Verification items for the finished model (mm, model axes). A direction names the side the tool comes from. Round coordinates to 2 decimals unless told otherwise and drop trailing zeros. Write each loop counter-clockwise with the first axis right and the second up, starting at its lowest first coordinate (ties: lowest second). Pieces come first, ordered by that corner, then holes. Notation, with made-up numbers: (64.5, -20.5) - (98.5, -20.5) arc R9 ccw to (98.5, -4.5) - close; hole circle Ø9 at (33, 44.5). An arc over 180 degrees is marked (long way). Answer as a JSON object with one key per item and string values.
```python
from build123d import *

# Parameters (mm, degrees)
BOSS_EXTRUDE1_DEPTH = 10
BOSS_EXTRUDE2_DEPTH = 130
FILLET1_R           = 0.8
SKETCH3_R           = 20
CUT_EXTRUDE1_DEPTH  = 5
CUT_EXTRUDE2_DEPTH  = 2


with BuildPart() as part:
    # Sketch1 → Boss-Extrude1 (new body)
    with BuildSketch(Plane(origin=(0, 0, 0), x_dir=(1, 0, 0), z_dir=(0, 1, 0))):
        Polygon((-35, 30), (-30, 35), (30, 35), (35, 30), (35, -30), (30, -35), (-30, -35), (-35, -30), align=None)
    extrude(amount=BOSS_EXTRUDE1_DEPTH)

    # Sketch2 → Boss-Extrude2 (add)
    with BuildSketch(Plane(origin=(0, 10, 0), x_dir=(1, 0, 0), z_dir=(0, 1, 0))):
        Polygon((-23.343145751, 19.343145751), (-19.343145751, 23.343145751), (-19.343145751, 27), (19.343145751, 27), (19.343145751, 23.343145751), (23.343145751, 19.343145751), (27, 19.343145751), (27, -19.343145751), (23.343145751, -19.343145751), (19.343145751, -23.343145751), (19.343145751, -27), (-19.343145751, -27), (-19.343145751, -23.343145751), (-23.343145751, -19.343145751), (-27, -19.343145751), (-27, 19.343145751), align=None)
    extrude(amount=BOSS_EXTRUDE2_DEPTH)

    # Fillet1
    fillet1_edges = [part.edges().sort_by_distance(p)[0] for p in [
        (27, 75, 19.343145751),
        (27, 75, -19.343145751),
        (23.343145751, 75, -19.343145751),
        (19.343145751, 75, -23.343145751),
        (19.343145751, 75, -27),
        (-19.343145751, 75, -27),
        (-19.343145751, 75, -23.343145751),
        (-23.343145751, 75, -19.343145751),
        (-27, 75, -19.343145751),
        (-27, 75, 19.343145751),
        (-23.343145751, 75, 19.343145751),
        (-19.343145751, 75, 23.343145751),
        (-19.343145751, 75, 27),
        (19.343145751, 75, 27),
        (19.343145751, 75, 23.343145751),
        (23.343145751, 75, 19.343145751),
    ]]
    fillet(fillet1_edges, radius=FILLET1_R)

    # Sketch3 → Cut-Extrude1 (cut)
    with BuildSketch(Plane(origin=(0, 140, 0), x_dir=(1, 0, 0), z_dir=(0, 1, 0))):
        Circle(SKETCH3_R)
    extrude(amount=-CUT_EXTRUDE1_DEPTH, mode=Mode.SUBTRACT)

    # Sketch5 → Cut-Extrude2 (cut)
    with BuildSketch(Plane(origin=(27, 0, 0), x_dir=(0, 0, -1), z_dir=(1, 0, 0))):
        Polygon((-4.112253732, 72.96796578), (3.887746268, 72.96796578), (-0.112253732, 67.96796578), align=None)
    extrude(amount=-CUT_EXTRUDE2_DEPTH, mode=Mode.SUBTRACT)


solid = part.part
```
Q1. Section check A-A, the plane x = 0. Record the cut outline in (y, z), then the cut area to 3 significant figures.
Geometry check:
{"outline": "(0, -35) - (10, -35) - (10, -27) - (140, -27) - (140, -20) - (135, -20) - (135, 20) - (140, 20) - (140, 27) - (10, 27) - (10, 35) - (0, 35) - close", "area": "7,520 mm2"}
Q2. Section check C-C, the plane z = -7. Record the cut outline in (x, y) (3 decimals).
Geometry check:
{"outline": "(-35, 0) - (35, 0) - (35, 10) - (27, 10) - (27, 140) - (18.735, 140) - (18.735, 135) - (-18.735, 135) - (-18.735, 140) - (-27, 140) - (-27, 10) - (-35, 10) - close"}
Q3. Material ranges on line 1 along Z through (x, y) = (0, 137.3); line 2 along Z through (x, y) = (4, 99.5), recorded low to high. Write a range as [from, to].
Geometry check:
{"line 1": "z = [-27, -20], [20, 27]", "line 2": "z = [-27, 27]"}
Q4. Set-up check for faces 1 (the flat face through (-21.368, 74.09, -21.318)), 2 (the flat face through (-27, 74, 0)), 3 (the flat face through (0, 74, 27)): record each of +Z, -Z, +X, -X, +Y, -Y from which the full face is reachable in a straight line by a thin tool's end or side.
Geometry check:
{"face 1": "-Z, -X, +Y", "face 2": "+Z, -Z, -X, +Y", "face 3": "+Z, +X, -X, +Y"}
Q5. Gauge pin test, flat ends, axial feed: P1, Ø20, axis at x = 1, z = 6, coming from the +Y side; P2, Ø10, axis at x = -12, y = 32.5, coming from the -Z side; P3, Ø18.5, axis at y = 76, z = -8, coming from the +X side. Record the tip position at first contact, or that the pin passes through.
Geometry check:
{"P1": "stops at y = 135", "P2": "stops at z = -27", "P3": "stops at x = 27"}
Q6. Release check for a two-part mould opening along Z. For faces 4 (the flat face through (35, 5, 0)), 5 (the flat face through (0, 135, 0)), 6 (the flat face through (-33, 5, -32)) record: released by +Z, released by -Z, zero draft, split by the parting line, or undercut.
Geometry check:
{"face 4": "zero draft", "face 5": "undercut", "face 6": "released by -Z"}
